Model file for the job. Use its own axes, mm. Face numbers are marked on the shaded views. Coordinates: 2 decimals unless noted, no trailing zeros. Order: outer loops, then holes, each group sorted by start corner. A loop starts at its lowest first (then second) coordinate and runs counter-clockwise, first axis right, second up.
from build123d import *

# Parameters (mm, degrees)
F0_R     = 37.5
F0_R_2   = 3
F0_R_3   = 5
F1_DEPTH = 6


# Not quite as in the source:
# - a feature names something its author has since deleted; it is built from what else it names


with BuildPart() as f1:
    # F0 (on Front) → F1 (new body)
    with BuildSketch(Plane.XZ):
        with Locations((0.1399259764, 30)):
            Circle(F0_R)
        with Locations((-31.9999092322, 29.8600740236)):
            Circle(F0_R_2, mode=Mode.SUBTRACT)
        with Locations((0.2798519529, -2.1398352087)):
            Circle(F0_R_2, mode=Mode.SUBTRACT)
        with Locations((0, 62.1398352087)):
            Circle(F0_R_2, mode=Mode.SUBTRACT)
        with Locations((0.1399259764, 30)):
            Circle(F0_R_3, mode=Mode.SUBTRACT)
        with Locations((32.2797611851, 30.1399259764)):
            Circle(F0_R_2, mode=Mode.SUBTRACT)
    extrude(amount=F1_DEPTH)


solid = f1.part
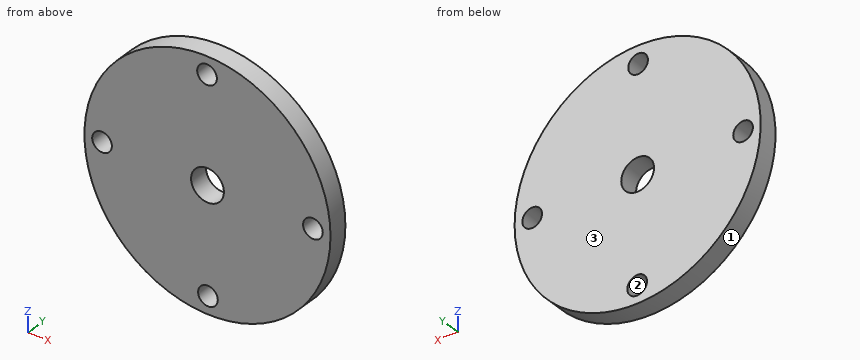
Q1. Cut at B-B, the plane z = 0. List the corners of the cut face in (x, y), plus the area to 3 significant figures.
Established:
outline: (-22.36, -6) - (-1.82, -6) - (-1.82, 0) - (-22.36, 0) - close; (2.38, -6) - (22.64, -6) - (22.64, 0) - (2.38, 0) - close
area: 245 mm2
Q2. Cut at A-A, the plane x = -31.5. List the corners of the cut face in (y, z), plus the area to 3 significant figures.
Established:
outline: (-6, 9.87) - (0, 9.87) - (0, 26.9) - (-6, 26.9) - close; (-6, 32.82) - (0, 32.82) - (0, 50.13) - (-6, 50.13) - close
area: 206 mm2
Q3. Cut at C-C, the plane y = -2.6. List the corners of the cut face in (x, z).
Established:
outline: circle Ø75 at (0.14, 30); hole circle Ø6 at (-32, 29.86); hole circle Ø10 at (0.14, 30); hole circle Ø6 at (0, 62.14); hole circle Ø6 at (0.28, -2.14); hole circle Ø6 at (32.28, 30.14)
Q4. Cut at D-D, the plane x = 1.5. List the corners of the cut face in (y, z), plus the area to 3 significant figures.
Established:
outline: (-6, -7.48) - (0, -7.48) - (0, -4.88) - (-6, -4.88) - close; (-6, 0.6) - (0, 0.6) - (0, 25.19) - (-6, 25.19) - close; (-6, 34.81) - (0, 34.81) - (0, 59.54) - (-6, 59.54) - close; (-6, 64.74) - (0, 64.74) - (0, 67.48) - (-6, 67.48) - close
area: 328 mm2
Q5. Mould opens along Z. For the marked faces 1, 2 and 3 say: pulls with the +Z half, pulls with the -Z half, needs draft (parallel to the pull), parting line crosses it, or undercut.
Established:
face 1: parting line crosses it
face 2: undercut
face 3: needs draft
Q6. Probe line 1 (X direction, y = -3.25, z = 31); line 2 (Z direction, x = -30, y = -2.5); line 3 (Z direction, x = 18.5, y = -5.45). List the from-to ranges inside material, lowest first.
Established:
line 1: x = -37.35 to -34.77, -29.22 to -4.76, 5.04 to 29.41, 35.15 to 37.63
line 2: z = 7.69 to 27.62, 32.1 to 52.31
line 3: z = -2.7 to 62.7
Q7. Drop flat-ended pins along their axis: P1, Ø8, axis at x = 0, z = 62.14, coming from the -Y side; P2, Ø3, axis at y = -1, z = 18, coming from the -X side; P3, Ø1.5, axis at x = -13.5, y = -3.5, coming from the -Z side; P4, Ø1.5, axis at y = -2, z = 54, coming from the +X side. Give the stop position or say it passes through.
Established:
P1: stops at y = -6
P2: stops at x = -35.86
P3: stops at z = -5.22
P4: stops at x = 29.56
